Verification items for the finished model (mm, model axes). A direction names the side the tool comes from. Coordinates: 2 decimals unless noted, no trailing zeros. Order: outer loops, then holes, each group sorted by start corner. A loop starts at its lowest first (then second) coordinate and runs counter-clockwise, first axis right, second up. Notation, with made-up numbers: M 6,-34 L 25,-34 A24 cw 25,-22 Z; hole C -8.75,-3.75 d2. An arc over 180 degrees is marked long. Return JSON: item names as keys, results as strings.
```python
from build123d import *

# Parameters (mm, degrees)
EXTRUDE_1_DEPTH = 6
FILLET_1_R      = 5
FILLET_2_R      = 3


with BuildPart() as part:
    # 草图1 → 凸台-拉伸1 (new body)
    with BuildSketch(Plane.XY):
        Polygon((-20, 0), (20, 0), (20, -20), (24, -20), (24, -18), (22, -18), (22, 2), (-22, 2), (-22, -18), (-24, -18), (-24, -20), (-20, -20), align=None)
    extrude(amount=EXTRUDE_1_DEPTH)

    # 圆角1
    # the kernel refuses this fillet: 5 mm, written as the material it adds along each edge
    with BuildSketch(Plane(origin=(22, -18, 0), x_dir=(1, 0, 0), z_dir=(0, 0, 1))) as fillet_1_piece_1:
        with BuildLine():
            CenterArc((5, 4), FILLET_1_R, 180, 53.130102354)
            Line((0, 4), (-0.1, 4))
            Line((-0.1, 4), (-0.1, 0))
            Line((-0.1, 0), (0, -0.1))
            ThreePointArc((0, -0.1), (1, -0.1), (1.94, -0.08))
            Line((1.94, -0.08), (2, 0))
        make_face()
    extrude(amount=6)
    with BuildSketch(Plane(origin=(-22, -18, 0), x_dir=(0, 1, 0), z_dir=(0, 0, 1))) as fillet_1_piece_2:
        with BuildLine():
            CenterArc((4, 5), FILLET_1_R, 216.869897646, 53.130102354)
            Line((0, 2), (-0.08, 1.94))
            ThreePointArc((-0.08, 1.94), (-0.1, 1), (-0.1, 0))
            Line((-0.1, 0), (0, -0.1))
            Line((0, -0.1), (4, -0.1))
            Line((4, -0.1), (4, 0))
        make_face()
    extrude(amount=6)

    # 圆角2
    fillet_2_edges = [part.edges().sort_by_distance(p)[0] for p in [
        (20, 0, 3),
        (-20, 0, 3),
        (-22, 2, 3),
        (22, 2, 3),
    ]]
    fillet(fillet_2_edges, radius=FILLET_2_R)


solid = part.part
```
Q1. Tool access check on faces 4 (the face through (22, -8, 3)), 5 (the face through (-22, -7, 3)), 6 (the face through (-24, -19, 3)), 7 (the face through (20, -11, 3)). Record the directions out of +Z, -Z, +X, -X, +Y, -Y that give a thin tool (end or side, any length) a straight path to the whole face; none if there is none.
Values:
{"face 4": "+Z, -Z, +X, +Y", "face 5": "+Z, -Z, -X, +Y", "face 6": "+Z, -Z, -X, +Y, -Y", "face 7": "+Z, -Z, -Y"}
Q2. Draft check along X on faces 1 (the face through (21.1, 1.14, 3.04)), 2 (the face through (-22, -20, 3)), 3 (the face through (0, 0, 3)). Enter one of: pulls with the +X half, pulls with the -X half, needs draft (parallel to the pull), parting line crosses it, or undercut.
Values:
{"face 1": "pulls with the +X half", "face 2": "needs draft", "face 3": "undercut"}
Q3. Go/stop test with flat-tipped pins: pin 1 (1.8 mm diameter, centred on y = -14.5, z = 2.5, fed in from +X); pin 2 (1.8 mm diameter, centred on y = -10.5, z = 4.5, fed in from -X). Record where each tip stops, or that it passes through.
Values:
{"pin 1": "x = 22.2", "pin 2": "x = -22"}
Q4. Cross-section at D-D, the plane y = -2. Record the boundary of the cut face in (x, z).
Values:
{"outline": "M -22,0 L -19.83,0 L -19.83,6 L -22,6 Z; M 19.83,0 L 22,0 L 22,6 L 19.83,6 Z"}
Q5. Cross-section at A-A, the plane y = -12. Record the boundary of the cut face in (x, z).
Values:
{"outline": "M -22,0 L -20,0 L -20,6 L -22,6 Z; M 20,0 L 22,0 L 22,6 L 20,6 Z"}
Q6. Material ranges on line 1 along X through (y, z) = (-2.75, 3.2); line 2 along Y through (x, z) = (-7.5, 1.35); line 3 along Y through (x, z) = (-19, 1.1), recorded low to high.
Values:
{"line 1": "-22 to -19.99, 19.99 to 22", "line 2": "0 to 2", "line 3": "-0.76 to 2"}
Q7. Cross-section at C-C, the plane x = 3.5. Record the boundary of the cut face in (y, z).
Values:
{"outline": "M 0,0 L 2,0 L 2,6 L 0,6 Z"}
Q8. Cross-section at B-B, the plane z = 4.7. Record the boundary of the cut face in (x, y), and give its area (3 significant figures).
Values:
{"outline": "M -24,-20 L -20,-20 L -20,-3 A3 cw -17,0 L 17,0 A3 cw 20,-3 L 20,-20 L 24,-20 L 24,-18 A5 cw 22,-14 L 22,-1 A3 ccw 19,2 L -19,2 A3 ccw -22,-1 L -22,-14 A5 cw -24,-18 Z", "area": "181 mm^2"}
